Model file for the job. Use its own axes, mm. Face numbers are marked on the shaded views. A direction names the side the tool comes from. Coordinates: 2 decimals unless noted, no trailing zeros. Loops run counter-clockwise (first coordinate to the right, second up) from the corner with the lowest first, then second, coordinate; pieces in that order, holes last. Notation, with made-up numbers: M 19,-40 L 45,-40 A26 cw 45,-4 Z; hole C -39.75,1.25 d7. An arc over 180 degrees is marked long. Write item = value, one per line. Start each with the question number.
from build123d import *

# Parameters (mm, degrees)
ESQUISSE2_R             = 2.75
ESQUISSE2_R_2           = 14.5
BOSS_EXTRU_1_DEPTH      = 32
BOSS_EXTRU_4_DEPTH      = 32
ENL_V_MAT_EXTRU_3_REACH = 88.563
ESQUISSE10_R            = 2.75
BOSS_EXTRU_6_DEPTH      = 20
ENL_V_MAT_EXTRU_4_REACH = 87.165
ENL_V_MAT_EXTRU_5_REACH = 91.18
ESQUISSE13_R            = 6


with BuildPart() as part:
    # Esquisse2 → Boss.-Extru.1 (new body)
    with BuildSketch(Plane.XY):
        with BuildLine():
            Line((20, 13.266499161), (20, -13.266499161))
            ThreePointArc((20, -13.266499161), (0, -24), (-20, -13.266499161))
            Line((-20, -13.266499161), (-20, 13.266499161))
            ThreePointArc((-20, 13.266499161), (0, 24), (20, 13.266499161))
        make_face()
        with Locations((0, 19)):
            Circle(ESQUISSE2_R, mode=Mode.SUBTRACT)
        with Locations((-13.435028843, 13.435028843)):
            Circle(ESQUISSE2_R, mode=Mode.SUBTRACT)
        with Locations((13.435028843, 13.435028843)):
            Circle(ESQUISSE2_R, mode=Mode.SUBTRACT)
        with Locations((0, -19)):
            Circle(ESQUISSE2_R, mode=Mode.SUBTRACT)
        with Locations((13.435028843, -13.435028843)):
            Circle(ESQUISSE2_R, mode=Mode.SUBTRACT)
        with Locations((-13.435028843, -13.435028843)):
            Circle(ESQUISSE2_R, mode=Mode.SUBTRACT)
        Circle(ESQUISSE2_R_2, mode=Mode.SUBTRACT)
    extrude(amount=BOSS_EXTRU_1_DEPTH)

    # Esquisse7 → Boss.-Extru.4 (add)
    with BuildSketch(Plane(origin=(0, 0, 0), x_dir=(-1, 0, 0), z_dir=(0, 0, -1))):
        with BuildLine():
            Line((-10, 63.000996071), (20, 13.266499161))
            ThreePointArc((20, 13.266499161), (0, 24), (-20, 13.266499161))
            Line((-20, 13.266499161), (-20, 36.422830435))
            Line((-20, 36.422830435), (-30, 53.000996071))
            Line((-30, 53.000996071), (-30, 63.000996071))
            Line((-30, 63.000996071), (-10, 63.000996071))
        make_face()
    extrude(amount=-BOSS_EXTRU_4_DEPTH)

    # Enlèv. mat.-Extru.3: up to this plane
    enl_v_mat_extru_3_end = Plane(origin=(10, 63.000996071, 102.523188973), z_dir=(-0.8562805371039014, 0.5165110277400223, 0))
    # Esquisse10 → Enlèv. mat.-Extru.3 (cut, up to the surface)
    with BuildSketch(Plane(origin=(30, 0, 0), x_dir=(0, 0, -1), z_dir=(1, 0, 0)), mode=Mode.PRIVATE) as enl_v_mat_extru_3_sk1:
        with Locations((-24.5, 58.000996071)):
            Circle(ESQUISSE10_R)
    enl_v_mat_extru_3_tool1 = split(extrude(enl_v_mat_extru_3_sk1.sketch, amount=-ENL_V_MAT_EXTRU_3_REACH, mode=Mode.PRIVATE), bisect_by=enl_v_mat_extru_3_end, keep=Keep.BOTH, mode=Mode.PRIVATE)
    add(enl_v_mat_extru_3_tool1.solids().sort_by_distance((30, 58.000996, 24.5))[0], mode=Mode.SUBTRACT)
    # Esquisse10 → Enlèv. mat.-Extru.3 (cut, up to the surface)
    with BuildSketch(Plane(origin=(30, 0, 0), x_dir=(0, 0, -1), z_dir=(1, 0, 0)), mode=Mode.PRIVATE) as enl_v_mat_extru_3_sk2:
        with Locations((-7.5, 58.000996071)):
            Circle(ESQUISSE10_R)
    enl_v_mat_extru_3_tool2 = split(extrude(enl_v_mat_extru_3_sk2.sketch, amount=-ENL_V_MAT_EXTRU_3_REACH, mode=Mode.PRIVATE), bisect_by=enl_v_mat_extru_3_end, keep=Keep.BOTH, mode=Mode.PRIVATE)
    add(enl_v_mat_extru_3_tool2.solids().sort_by_distance((30, 58.000996, 7.5))[0], mode=Mode.SUBTRACT)

    # Esquisse11 → Boss.-Extru.6 (add)
    with BuildSketch(Plane(origin=(30, 0, 0), x_dir=(0, 0, -1), z_dir=(1, 0, 0))):
        Polygon((-32, 63.000996071), (0, 63.000996071), (-3.5, 73.000996071), (-32, 63.500996071), align=None)
    extrude(amount=-BOSS_EXTRU_6_DEPTH)

    # Esquisse12 → Enlèv. mat.-Extru.4 (cut, up to next)
    with BuildSketch(Plane(origin=(0, 0, 0), x_dir=(-1, 0, 0), z_dir=(0, 0, -1)), mode=Mode.PRIVATE) as enl_v_mat_extru_4_sk1:
        Polygon((-10, 63.000996071), (-17.962764916, 73.000996071), (-10, 73.000996071), align=None)
    enl_v_mat_extru_4_tool1 = extrude(enl_v_mat_extru_4_sk1.sketch, amount=-ENL_V_MAT_EXTRU_4_REACH, mode=Mode.PRIVATE) & part.part
    add(enl_v_mat_extru_4_tool1.solids().sort_by_distance((12.654255, 69.667663, 0))[0], mode=Mode.SUBTRACT)

    # Esquisse13 → Enlèv. mat.-Extru.5 (cut, up to next)
    with BuildSketch(Plane(origin=(20, 0, 0), x_dir=(0, 0, -1), z_dir=(1, 0, 0)), mode=Mode.PRIVATE) as enl_v_mat_extru_5_sk1:
        with Locations((-7.5, 58.000996071)):
            Circle(ESQUISSE13_R)
    enl_v_mat_extru_5_tool1 = extrude(enl_v_mat_extru_5_sk1.sketch, amount=-ENL_V_MAT_EXTRU_5_REACH, mode=Mode.PRIVATE) & part.part
    # Esquisse13 → Enlèv. mat.-Extru.5 (cut, up to next)
    with BuildSketch(Plane(origin=(20, 0, 0), x_dir=(0, 0, -1), z_dir=(1, 0, 0)), mode=Mode.PRIVATE) as enl_v_mat_extru_5_sk2:
        with Locations((-24.5, 58.000996071)):
            Circle(ESQUISSE13_R)
    enl_v_mat_extru_5_tool2 = extrude(enl_v_mat_extru_5_sk2.sketch, amount=-ENL_V_MAT_EXTRU_5_REACH, mode=Mode.PRIVATE) & part.part
    add(enl_v_mat_extru_5_tool1.solids().sort_by_distance((20, 58.000996, 7.5))[0], mode=Mode.SUBTRACT)
    add(enl_v_mat_extru_5_tool2.solids().sort_by_distance((20, 58.000996, 24.5))[0], mode=Mode.SUBTRACT)


solid = part.part
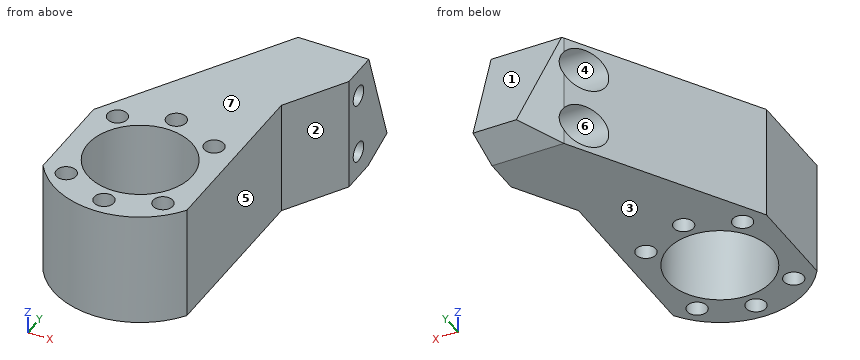
Item 1: Cut at B-B (z = 24). Give the number of separate pieces and of enclosed holes in the cut face, plus the area to 3 significant figures.
Item 2: 3-axis set-ups, long thin cutter, end or side, ignore diameter. For the marked faces 5, 6 and 7: which of +Z, -Z, +X, -X, +Y, -Y reach the whole face in a straight line?
Item 3: Pull direction Z, two halves, no side cores. Call the marked faces 1, 2, 3 and 4: +Z half, -Z half, draft (parallel to the pull), parting line (faces both ways), or undercut.
Item 4: Pin check, flat tips, straight feed: pin 1 Ø4.5 at (x, y) = (0, -19) entering from +Z; pin 2 Ø6 at (x, z) = (-13, 28) entering from -Y; pin 3 Ø12 at (x, y) = (12, -6.5) entering from -Z; pin 4 Ø6 at (x, z) = (-0.5, 18.5) entering from +Y. Stop position of each tip, or through.
Item 5: Cut at D-D (x = -8). Give the cut face in (y, z), plus the area to 3 significant figures.
Item 6: Probe L1, parallel to Z at x = 15, y = 63; L2, parallel to Y at x = 2, z = 18; L3, parallel to Y at x = -15, z = 17 (3 decimals). List the from-to ranges inside material, lowest first.
Item 7: Cut at A-A (y = -19). Give the cut face in (x, z).
Item 8: Cut at C-C (x = 23). Give the cut face in (y, z), plus the area to 3 significant figures.
Reported:
q1.separate_pieces = 2
q1.enclosed_holes = 7
q1.area = 1,840 mm^2
q2.face_5 = +Z, -Z, +X, -Y
q2.face_6 = -X
q2.face_7 = +Z, +X, -X, +Y, -Y
q3.face_1 = +Z half
q3.face_2 = draft
q3.face_3 = -Z half
q3.face_4 = undercut
q4.pin_1 = through
q4.pin_2 = -21.82
q4.pin_3 = 0
q4.pin_4 = 50.57
q5.outline = M -22.63,0 L -12.09,0 L -12.09,32 L -22.63,32 Z; M 12.09,0 L 33.16,0 L 33.16,32 L 12.09,32 Z
q5.area = 1,010 mm^2
q6.L1 = 0 to 4.18, 10.82 to 21.18, 27.82 to 32
q6.L2 = -23.92 to -20.89, -17.11 to -14.36, 14.36 to 17.11, 20.89 to 49.74
q6.L3 = -18.735 to -15.696, -11.174 to 11.174, 15.696 to 21.556
q7.outline = M -14.66,0 L -2.75,0 L -2.75,32 L -14.66,32 Z; M 2.75,0 L 14.66,0 L 14.66,32 L 2.75,32 Z
q8.outline = M 41.4,0 L 63,0 L 73,3.5 L 63.5,32 L 41.4,32 Z; hole C 58,7.5 d5.5; hole C 58,24.5 d5.5
q8.area = 811 mm^2
